Input: part model. Units: mm. Frame: model coordinates. Face numbers are marked on the shaded views. A direction names the side the tool comes from. Coordinates: 2 decimals unless noted, no trailing zeros. Loops run counter-clockwise (first coordinate to the right, second up) from the corner with the lowest first, then second, coordinate; pieces in that order, holes last.
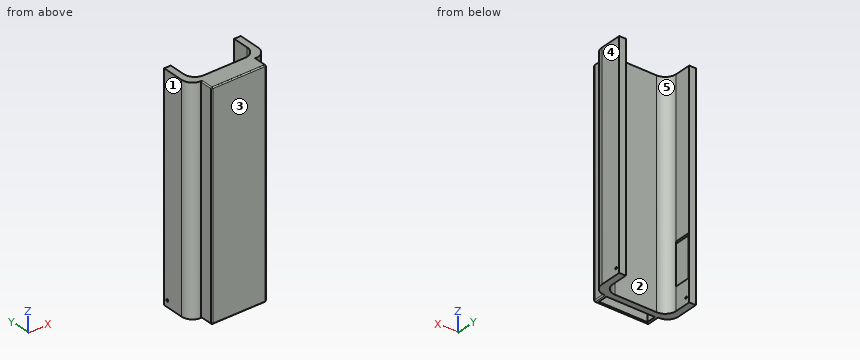
```python
from build123d import *

# Parameters (mm, degrees)
BOSS_EXTRUDE1_DEPTH      = 200
FILLET1_R                = 10
SKETCH12_W               = 38
SKETCH12_H               = 17.8
CUT_EXTRUDE9_DEPTH       = 2
BOSS_EXTRUDE2_DEPTH      = 200
FILLET4_R                = 1
SKETCH17_W               = 44.239510651
SKETCH17_H               = 8.731521098
CUT_EXTRUDE11_DEPTH      = 193
CUT_EXTRUDE12_DEPTH      = 215.329567289
CUT_EXTRUDE12_DEPTH_BACK = 215.329567289
SKETCH20_R               = 1


with BuildPart() as part:
    # Sketch1 → Boss-Extrude1 (new body)
    with BuildSketch(Plane.XY):
        Polygon((-30.275246352, -0.908779536), (-30.275246352, -25.913082449), (27.724753648, -25.913082449), (27.724753648, -0.908779536), (33.724753648, -0.908779536), (33.724753648, -30.908779536), (-36.275246352, -30.908779536), (-36.275246352, -0.908779536), align=None)
    extrude(amount=BOSS_EXTRUDE1_DEPTH)

    # Fillet1
    fillet1_edges = [part.edges().sort_by_distance(p)[0] for p in [
        (-30.275246352, -25.913082449, 100),
        (27.724753648, -25.913082449, 100),
        (33.724753648, -30.908779536, 100),
        (-36.275246352, -30.908779536, 100),
    ]]
    fillet(fillet1_edges, radius=FILLET1_R)

    # Sketch12 → Cut-Extrude9 (cut)
    with BuildSketch(Plane(origin=(-30.275246352, 0, 0), x_dir=(0, 0, -1), z_dir=(1, 0, 0))):
        with Locations((-39.87, -10.658779536)):
            Rectangle(SKETCH12_W, SKETCH12_H)
    extrude(amount=-CUT_EXTRUDE9_DEPTH, mode=Mode.SUBTRACT)

    # Sketch15 → Boss-Extrude2 (add)
    with BuildSketch(Plane.XY):
        Polygon((-26.275246352, -30.908779536), (-26.275246352, -42.908779536), (23.724753648, -42.908779536), (23.724753648, -30.908779536), (20.724753648, -30.908779536), (-23.275246352, -30.908779536), align=None)
    extrude(amount=BOSS_EXTRUDE2_DEPTH)

    # Fillet4
    fillet4_edges = [part.edges().sort_by_distance(p)[0] for p in [
        (-26.275246352, -36.908779536, 0),
        (-26.275246352, -42.908779536, 100),
        (-1.275246352, -42.908779536, 0),
        (23.724753648, -42.908779536, 100),
        (23.724753648, -36.908779536, 0),
        (-26.275246352, -36.908779536, 200),
        (-1.275246352, -42.908779536, 200),
        (23.724753648, -36.908779536, 200),
    ]]
    fillet(fillet4_edges, radius=FILLET4_R)

    # Sketch17 → Cut-Extrude11 (cut)
    with BuildSketch(Plane(origin=(0, 0, 0), x_dir=(-1, 0, 0), z_dir=(0, 0, -1))):
        with Locations((1.300040019, -36.058148136)):
            Rectangle(SKETCH17_W, SKETCH17_H)
    extrude(amount=-CUT_EXTRUDE11_DEPTH, mode=Mode.SUBTRACT)

    # Sketch20 → Cut-Extrude12 (cut, two sides: drawn at the far end of the back side and taken through both)
    with BuildSketch(Plane.ZY.offset(-27.724753648).offset(-CUT_EXTRUDE12_DEPTH_BACK)):
        with Locations(Location((5.712078597, -4.528347047, 0), (0, 0, 270))):
            Circle(SKETCH20_R)
    extrude(amount=CUT_EXTRUDE12_DEPTH + CUT_EXTRUDE12_DEPTH_BACK, mode=Mode.SUBTRACT)


solid = part.part
```
Item 1: Reachability of the marked faces 1 and 2 from +Z, -Z, +X, -X, +Y, -Y: full face, straight path, thin tool, end or side. Return the list, or none.
Result:
face 1: +Z, -Z, -X, +Y, -Y
face 2: +Z, -Z, +Y
Item 2: Section query D-D (z = 29.5). Output: boundary loops of the cut face in (x, y), then the cut area to 3 significant figures.
Result:
outline: (-36.28, -20.91) arc R10 ccw to (-26.28, -30.91) - (-26.28, -41.91) arc R1 ccw to (-25.28, -42.91) - (22.72, -42.91) arc R1 ccw to (23.72, -41.91) - (23.72, -30.91) arc R10 ccw to (33.72, -20.91) - (33.72, -0.91) - (27.72, -0.91) - (27.72, -15.91) arc R10 cw to (17.72, -25.91) - (-20.28, -25.91) arc R10 cw to (-30.28, -15.91) - (-30.28, -19.56) - (-32.28, -19.56) - (-32.28, -1.76) - (-30.28, -1.76) - (-30.28, -0.91) - (-36.28, -0.91) - close; hole (-23.42, -40.42) - (20.82, -40.42) - (20.82, -31.69) - (-23.42, -31.69) - close
area: 827 mm2
Item 3: Section query B-B (y = -34.5). Output: boundary loops of the cut face in (x, z), then the cut area to 3 significant figures.
Result:
outline: (-26.28, 1) arc R1 ccw to (-25.28, 0) - (-23.42, 0) - (-23.42, 193) - (20.82, 193) - (20.82, 0) - (22.72, 0) arc R1 ccw to (23.72, 1) - (23.72, 199) arc R1 ccw to (22.72, 200) - (-25.28, 200) arc R1 ccw to (-26.28, 199) - close
area: 1,460 mm2
Item 4: Contact query for flat-ended pins moving along their axis: P1, Ø2, axis at x = -31.5, y = -9, coming from the -Z side; P2, Ø1.2, axis at y = -4.53, z = 5.71, coming from the -X side; P3, Ø2.5, axis at y = -38, z = 71.5, coming from the -X side; P4, Ø5.5, axis at y = -34, z = 72.5, coming from the +X side. Output: stop coordinate, or through.
Result:
P1: stops at z = 0
P2: passes through
P3: stops at x = -26.28
P4: stops at x = 23.72
Item 5: Line query: L1, parallel to X at y = -15.5, z = 36.5; L2, parallel to Y at x = 1, z = 141.5; L3, parallel to X at y = -7.5, z = 131.5. Output: solid intervals per line, ascending.
Result:
L1: x = -36.28 to -32.28, 27.72 to 33.72
L2: y = -42.91 to -40.42, -31.69 to -25.91
L3: x = -36.28 to -30.28, 27.72 to 33.72
Item 6: Mould query, pull axis X, two halves, no side actions, for the marked faces 3, 4 and 5. Classes: +X half, -X half, draft (parallel to the pull), parting line (faces both ways), or undercut.
Result:
face 3: draft
face 4: +X half
face 5: undercut
Item 7: Section query A-A (z = 124). Output: boundary loops of the cut face in (x, y), then the cut area to 3 significant figures.
Result:
outline: (-36.28, -20.91) arc R10 ccw to (-26.28, -30.91) - (-26.28, -41.91) arc R1 ccw to (-25.28, -42.91) - (22.72, -42.91) arc R1 ccw to (23.72, -41.91) - (23.72, -30.91) arc R10 ccw to (33.72, -20.91) - (33.72, -0.91) - (27.72, -0.91) - (27.72, -15.91) arc R10 cw to (17.72, -25.91) - (-20.28, -25.91) arc R10 cw to (-30.28, -15.91) - (-30.28, -0.91) - (-36.28, -0.91) - close; hole (-23.42, -40.42) - (20.82, -40.42) - (20.82, -31.69) - (-23.42, -31.69) - close
area: 863 mm2
Item 8: Section query C-C (x = 12.5). Output: boundary loops of the cut face in (y, z).
Result:
outline: (-42.91, 1) arc R1 ccw to (-41.91, 0) - (-40.42, 0) - (-40.42, 193) - (-31.69, 193) - (-31.69, 0) - (-25.91, 0) - (-25.91, 200) - (-41.91, 200) arc R1 ccw to (-42.91, 199) - close
